from build123d import *

# Parameters (mm, degrees)
SKETCH1_W           = 29.9
SKETCH1_H           = 11
BOSS_EXTRUDE1_DEPTH = 5.6
SKETCH2_R           = 4
BOSS_EXTRUDE2_DEPTH = 2
CUT_EXTRUDE1_START  = -5.6
CUT_EXTRUDE1_DEPTH  = 5.6
SKETCH5_R           = 3.25
BOSS_EXTRUDE3_DEPTH = 1.5
SKETCH6_R           = 1.45
BOSS_EXTRUDE4_DEPTH = 4.5
SKETCH7_W           = 3.4
SKETCH7_H           = 6.5
CUT_EXTRUDE2_DEPTH  = 5.6
FILLET2_R           = 4
SKETCH8_R           = 0.5
BOSS_EXTRUDE5_DEPTH = 5.6
FILLET3_R           = 0.5
SKETCH9_R           = 0.95
CUT_EXTRUDE3_DEPTH  = 4.5
FILLET5_R           = 1
SKETCH10_W          = 10.9
SKETCH10_H          = 1.5
CUT_EXTRUDE4_DEPTH  = 5.6
FILLET6_R           = 1
FILLET7_R           = 1
FILLET8_R           = 0.2
SKETCH11_W          = 9.2
SKETCH11_H          = 3.7
CUT_EXTRUDE5_DEPTH  = 1
FILLET9_R           = 2
BOSS_EXTRUDE6_DEPTH = 0.4
FILLET10_R          = 1


with BuildPart() as part:
    # Sketch1 → Boss-Extrude1 (new body)
    with BuildSketch(Plane.XY):
        with Locations((44.023400912, -0.002506593)):
            Rectangle(SKETCH1_W, SKETCH1_H)
    extrude(amount=BOSS_EXTRUDE1_DEPTH)

    # Sketch2 → Boss-Extrude2 (add)
    with BuildSketch(Plane(origin=(0, 0, 0), x_dir=(-1, 0, 0), z_dir=(0, 0, -1))):
        with Locations((-33.073400912, -1.502506593)):
            Circle(SKETCH2_R)
    extrude(amount=BOSS_EXTRUDE2_DEPTH)

    # Sketch4 → Cut-Extrude1 (cut)
    with BuildSketch(Plane(origin=(0, 0, 0), x_dir=(-1, 0, 0), z_dir=(0, 0, -1)).offset(CUT_EXTRUDE1_START)):
        with BuildLine():
            Line((-29.073400912, -1.502506593), (-29.073400912, -5.502506593))
            Line((-29.073400912, -5.502506593), (-33.073400912, -5.502506593))
            ThreePointArc((-33.073400912, -5.502506593), (-30.244973787, -4.330933718), (-29.073400912, -1.502506593))
        make_face()
    extrude(amount=CUT_EXTRUDE1_DEPTH, mode=Mode.SUBTRACT)

    # Sketch5 → Boss-Extrude3 (add)
    with BuildSketch(Plane.XY.offset(5.6)):
        with Locations((51.073400912, -1.002506593)):
            Circle(SKETCH5_R)
    extrude(amount=BOSS_EXTRUDE3_DEPTH)

    # Sketch6 → Boss-Extrude4 (add)
    with BuildSketch(Plane.XY.offset(7.1)):
        with Locations((51.073400912, -1.002506593)):
            Circle(SKETCH6_R)
    extrude(amount=BOSS_EXTRUDE4_DEPTH)

    # Sketch7 → Cut-Extrude2 (cut)
    with BuildSketch(Plane.XY.offset(5.6)):
        with Locations((57.273400912, -2.252506593)):
            Rectangle(SKETCH7_W, SKETCH7_H)
    extrude(amount=-CUT_EXTRUDE2_DEPTH, mode=Mode.SUBTRACT)

    # Fillet2
    fillet2_edges = [part.edges().sort_by_distance(p)[0] for p in [
        (55.573400912, -5.502506593, 2.8),
    ]]
    fillet(fillet2_edges, radius=FILLET2_R)

    # Sketch8 → Boss-Extrude5 (add)
    with BuildSketch(Plane.XY.offset(5.6)):
        with Locations((52.073400912, 5.497493407)):
            Circle(SKETCH8_R)
    extrude(amount=-BOSS_EXTRUDE5_DEPTH)

    # Fillet3
    fillet3_edges = [part.edges().sort_by_distance(p)[0] for p in [
        (52.573400912, 5.497493407, 2.8),
        (51.573400912, 5.497493407, 2.8),
    ]]
    fillet(fillet3_edges, radius=FILLET3_R)

    # Sketch9 → Cut-Extrude3 (cut)
    with BuildSketch(Plane.XZ.offset(-0.997493407)):
        with Locations((56.973400912, 1.5)):
            Circle(SKETCH9_R)
    extrude(amount=-CUT_EXTRUDE3_DEPTH, mode=Mode.SUBTRACT)

    # Fillet5
    fillet5_edges = [part.edges().sort_by_distance(p)[0] for p in [
        (58.973400912, 5.497493407, 2.8),
    ]]
    fillet(fillet5_edges, radius=FILLET5_R)

    # Sketch10 → Cut-Extrude4 (cut)
    with BuildSketch(Plane.XY.offset(5.6)):
        with Locations((34.523400912, 4.747493407)):
            Rectangle(SKETCH10_W, SKETCH10_H)
    extrude(amount=-CUT_EXTRUDE4_DEPTH, mode=Mode.SUBTRACT)

    # Fillet6
    fillet6_edges = [part.edges().sort_by_distance(p)[0] for p in [
        (29.073400912, 3.997493407, 2.8),
    ]]
    fillet(fillet6_edges, radius=FILLET6_R)

    # Fillet7
    fillet7_edges = [part.edges().sort_by_distance(p)[0] for p in [
        (39.973400912, 3.997493407, 2.8),
    ]]
    fillet(fillet7_edges, radius=FILLET7_R)

    # Fillet8
    fillet8_edges = [part.edges().sort_by_distance(p)[0] for p in [
        (39.973400912, 5.497493407, 2.8),
    ]]
    fillet(fillet8_edges, radius=FILLET8_R)

    # Sketch11 → Cut-Extrude5 (cut)
    with BuildSketch(Plane(origin=(0, 0, 0), x_dir=(-1, 0, 0), z_dir=(0, 0, -1))):
        with Locations((-43.323400912, 3.647493407)):
            Rectangle(SKETCH11_W, SKETCH11_H)
    extrude(amount=-CUT_EXTRUDE5_DEPTH, mode=Mode.SUBTRACT)

    # Fillet9
    fillet9_edges = [part.edges().sort_by_distance(p)[0] for p in [
        (47.923400912, 1.797493407, 0.5),
    ]]
    fillet(fillet9_edges, radius=FILLET9_R)

    # Sketch12 → Boss-Extrude6 (add)
    with BuildSketch(Plane(origin=(0, 0, 0), x_dir=(-1, 0, 0), z_dir=(0, 0, -1))):
        with BuildLine():
            Line((-37.073400912, -1.502506593), (-38.744359598, -1.502506593))
            Line((-38.744359598, -1.502506593), (-38.744359598, -4.080351874))
            Line((-38.744359598, -4.080351874), (-36.537502527, -3.502506593))
            ThreePointArc((-36.537502527, -3.502506593), (-36.937104217, -2.537782773), (-37.073400912, -1.502506593))
        make_face()
    extrude(amount=BOSS_EXTRUDE6_DEPTH)

    # Fillet10
    fillet10_edges = [part.edges().sort_by_distance(p)[0] for p in [
        (38.744359598, -1.502506593, -0.2),
        (38.744359598, -4.080351874, -0.2),
    ]]
    fillet(fillet10_edges, radius=FILLET10_R)


solid = part.part
Can you work these out from the model? Positions are in its coordinate system, mm. A direction names the side the tool comes from. Coordinates: 2 decimals unless noted, no trailing zeros. Write each loop counter-clockwise with the first axis right and the second up, starting at its lowest first coordinate (ties: lowest second). Pieces come first, ordered by that corner, then holes. Notation, with made-up numbers: M 22.25,16.25 L 43.25,16.25 A29 ccw 43.25,38.25 Z; hole C -38.75,74.25 d5. An arc over 180 degrees is marked long. Use one line per item in the form item = value.
Q1. If we section it at C-C (y = -0.5): Write out the boundary of the cut face in (x, z), then the cut area to 3 significant figures.
Model answer:
outline = M 29.07,0 L 29.2,0 L 29.2,-2 L 36.95,-2 L 36.95,0 L 55.57,0 L 55.57,5.6 L 54.28,5.6 L 54.28,7.1 L 52.43,7.1 L 52.43,11.6 L 49.71,11.6 L 49.71,7.1 L 47.86,7.1 L 47.86,5.6 L 29.07,5.6 Z
area = 186 mm^2
Q2. If we section it at A-A (z = 1.5): Write out the boundary of the cut face in (x, y), then the cut area to 3 significant figures.
Model answer:
outline = M 29.07,-1.5 A4 ccw 33.07,-5.5 L 51.57,-5.5 A4 ccw 55.57,-1.5 L 55.57,1 L 56.02,1 L 56.02,5.5 L 52.94,5.5 A0.5 cw 52.51,5.75 A0.5 ccw 51.64,5.75 A0.5 cw 51.21,5.5 L 40.17,5.5 A0.2 ccw 39.97,5.3 L 39.97,5 A1 cw 38.97,4 L 30.07,4 A1 ccw 29.07,3 Z; M 57.92,1 L 58.97,1 L 58.97,4.5 A1 ccw 57.97,5.5 L 57.92,5.5 Z
area = 275 mm^2
Q3. We'd pull the mould along X, two halves only. Please class faces 1 (the flat face through (38.723, 2.9, 0.5)), 2 (the cylindrical face through (47.827, -0.86, 6.339)), 3 (the flat face through (46, 5.497, 3)): +X half, -X half, draft (parallel to the pull), parting line (faces both ways), or undercut.
Model answer:
face_1 = undercut
face_2 = parting line
face_3 = draft
Q4. If we section it at D-D (z = 10.75): Write out the boundary of the cut face in (x, y), then the cut area to 3 significant figures.
Model answer:
outline = C 51.07,-1 d2.9
area = 6.61 mm^2
Q5. I need wall thicknesses on line 1 along Z through (x, y) = (41.5, -1); line 2 along Y through (x, z) = (33.25, 0.25); line 3 along Z through (x, y) = (36, 0.25). Which ranges of each line are inside material? Lowest first, please. Write a range as from..to.
Model answer:
line_1 = 0..5.6
line_2 = -5.5..4
line_3 = -2..5.6
Q6. For faces 4 (the flat face through (43, 4, 1)), 5 (the cylindrical face through (38.459, -1.803, -0.203)), 6 (the flat face through (57, 0.997, 3)), which set-ups out of +Z, -Z, +X, -X, +Y, -Y let a thin tool reach every point of the face, with its end or its side?
Model answer:
face_4 = -Z, +Y
face_5 = -Z, +X, +Y
face_6 = +Z, -Z, +X, -Y
Q7. If we section it at B-B (x = 32.25): Write out the boundary of the cut face in (y, z).
Model answer:
outline = M -5.42,-2 L 2.41,-2 L 2.41,0 L 4,0 L 4,5.6 L -5.42,5.6 Z
Q8. For P1, Ø6, axis at x = 41.5, y = 2, coming from the +Z side; P2, Ø1.7, axis at x = 46.5, z = 1.5, coming from the +Y side; P3, Ø1.9, axis at x = 43, y = 3.5, coming from the -Z side, each with a flat end and sliding along its axis, tell me the tip position at first contact or that it passes through.
Model answer:
P1 = 5.6
P2 = 5.5
P3 = 1
